```python
from build123d import *

# Parameters (mm, degrees)
EXTRUDE_1_DEPTH        = 150
SKETCH_3_R             = 2.25
CUT_EXTRUDE_1_DEPTH    = 20
PATTERN_LINEAR_1_COUNT = 2
PATTERN_LINEAR_1_PITCH = 75


with BuildPart() as part:
    # 草图2 → 凸台-拉伸1 (new body)
    with BuildSketch(Plane.XY):
        with BuildLine():
            Line((2.35, -4.413332075), (7.752951986, -16))
            Line((7.752951986, -16), (17.5, -16))
            Line((17.5, -16), (17.5, -20))
            Line((17.5, -20), (-17.5, -20))
            Line((-17.5, -20), (-17.5, -16))
            Line((-17.5, -16), (-7.752951986, -16))
            Line((-7.752951986, -16), (-2.35, -4.413332075))
            ThreePointArc((-2.35, -4.413332075), (0, -5), (2.35, -4.413332075))
        make_face()
    extrude(amount=-EXTRUDE_1_DEPTH)

    # 草图3 → 切除-拉伸1 (cut)
    with BuildSketch(Plane(origin=(0, 0, 0), x_dir=(1, 0, 0), z_dir=(0, 1, 0))):
        with Locations(Location((12.5, 37.5, 0), (0, 0, 270))):
            Circle(SKETCH_3_R)
        with Locations(Location((-12.5, 37.5, 0), (0, 0, 270))):
            Circle(SKETCH_3_R)
    cut_extrude_1 = extrude(amount=-CUT_EXTRUDE_1_DEPTH, mode=Mode.SUBTRACT)

    # 草图4 → 切除-旋转1 (revolve, cut)
    with BuildSketch(Plane.XY.offset(-37.5), mode=Mode.PRIVATE) as cut_revolve_1_sk:
        Polygon((-2.25, -4.465142775), (-2.25, -13.815142775), (-3.15, -13.815142775), (-3.15, -20), (0, -20), (0, -4.465142775), align=None)
    cut_revolve_1 = revolve(cut_revolve_1_sk.sketch.rotate(Axis((0, -20, -37.5), (0, 1, 0)), 180), axis=Axis((0, -20, -37.5), (0, 1, 0)), mode=Mode.SUBTRACT)

    # 阵列(线性)1: 切除-拉伸1, 切除-旋转1 ×2
    with Locations(*[(0, 0, -i * PATTERN_LINEAR_1_PITCH) for i in range(1, PATTERN_LINEAR_1_COUNT)]):
        add(cut_extrude_1, mode=Mode.SUBTRACT)
        add(cut_revolve_1, mode=Mode.SUBTRACT)


solid = part.part
```
The listing builds one solid part. Answer for the finished solid, in the listing's coordinates (mm). A direction names the side the tool comes from. Round coordinates to 2 decimals unless told otherwise and drop trailing zeros. Loops run counter-clockwise (first coordinate to the right, second up) from the corner with the lowest first, then second, coordinate; pieces in that order, holes last. Notation, with made-up numbers: (72.5, 88.5) -> (89.5, 88.5) arc R6 cw to (89.5, 97.5) -> close; hole circle Ø1 at (23.5, 11). An arc over 180 degrees is marked (long way). Use one line per item in the form item = value.
1. Find the intervals of material crossed by probe 1 along X at (y, z) = (-18.1, -37.5); probe 2 along Z at (x, y) = (0, -17.25); probe 3 along Z at (x, y) = (0, -11.25), in increasing order. Write a range as [from, to].
Answer key:
probe_1 = [-17.5, -14.75], [-10.25, -3.15], [3.15, 10.25], [14.75, 17.5]
probe_2 = [-150, -115.65], [-109.35, -40.65], [-34.35, 0]
probe_3 = [-150, -114.75], [-110.25, -39.75], [-35.25, 0]
2. For a pull along X with two mould halves and no side action, classify faces 4 (the flat face through (1, -13.815, -115)), 5 (the flat face through (1, -13.815, -40)), 6 (the flat face through (13, -16, -74)), 7 (the flat face through (-5.09, -10.29, -73.95)) as released by +X, released by -X, zero draft, split by the parting line, or undercut.
Answer key:
face_4 = undercut
face_5 = undercut
face_6 = zero draft
face_7 = released by -X
3. The part is cut by section B-B on z = -37.5. Determine the outline of the cut face in (x, y).
Answer key:
outline = (-17.5, -20) -> (-14.75, -20) -> (-14.75, -16) -> (-17.5, -16) -> close; (-10.25, -20) -> (-3.15, -20) -> (-3.15, -13.82) -> (-2.25, -13.82) -> (-2.25, -4.47) arc R5 cw to (-2.35, -4.41) -> (-7.75, -16) -> (-10.25, -16) -> close; (2.25, -13.82) -> (3.15, -13.82) -> (3.15, -20) -> (10.25, -20) -> (10.25, -16) -> (7.75, -16) -> (2.35, -4.41) arc R5 cw to (2.25, -4.47) -> close; (14.75, -20) -> (17.5, -20) -> (17.5, -16) -> (14.75, -16) -> close
4. The part is cut by section C-C on y = -17.25. Determine the outline of the cut face in (x, z).
Answer key:
outline = (-17.5, -150) -> (17.5, -150) -> (17.5, 0) -> (-17.5, 0) -> close; hole circle Ø4.5 at (-12.5, -112.5); hole circle Ø4.5 at (-12.5, -37.5); hole circle Ø6.3 at (0, -112.5); hole circle Ø6.3 at (0, -37.5); hole circle Ø4.5 at (12.5, -112.5); hole circle Ø4.5 at (12.5, -37.5)
5. The part is cut by section A-A on x = 0. Determine the outline of the cut face in (y, z).
Answer key:
outline = (-20, -150) -> (-5, -150) -> (-5, -114.75) -> (-13.82, -114.75) -> (-13.82, -115.65) -> (-20, -115.65) -> close; (-20, -109.35) -> (-13.82, -109.35) -> (-13.82, -110.25) -> (-5, -110.25) -> (-5, -39.75) -> (-13.82, -39.75) -> (-13.82, -40.65) -> (-20, -40.65) -> close; (-20, -34.35) -> (-13.82, -34.35) -> (-13.82, -35.25) -> (-5, -35.25) -> (-5, 0) -> (-20, 0) -> close
6. A tool of negligible diameter and unlimited length cuts with its end or side. For faces 1 (the cylindrical face through (-0.488, -9.206, -110.304)), 2 (the cylindrical face through (-0.41, -16.951, -115.623)), 3 (the flat face through (-13, -16, -74)), from which of +Z, -Z, +X, -X, +Y, -Y can it reach the whole face along a straight path? Write none if from no direction.
Answer key:
face_1 = +Y, -Y
face_2 = -Y
face_3 = +Z, -Z, -X, +Y
7. Flat-ended cylindrical pins translate along their axes: pin 1 Ø1.5 at (x, z) = (-6, -102) entering from +Y; pin 2 Ø8 at (x, z) = (0, -112.5) entering from +Y; pin 3 Ø6 at (x, z) = (0, -112.5) entering from -Y. Find the tip coordinate at first contact, or state that the pin passes through.
Answer key:
pin_1 = -10.63
pin_2 = -4.41
pin_3 = -13.82
8. The part is cut by section D-D on z = -88.5. Determine the outline of the cut face in (x, y), and give its area (3 significant figures).
Answer key:
outline = (-17.5, -20) -> (17.5, -20) -> (17.5, -16) -> (7.75, -16) -> (2.35, -4.41) arc R5 cw to (-2.35, -4.41) -> (-7.75, -16) -> (-17.5, -16) -> close
area = 255 mm²
